Can you work these out from the model? Positions are in its coordinate system, mm. A direction names the side the tool comes from. Round coordinates to 2 decimals unless told otherwise and drop trailing zeros. Loops run counter-clockwise (first coordinate to the right, second up) from the corner with the lowest first, then second, coordinate; pieces in that order, holes last.
from build123d import *

# Parameters (mm, degrees)
SKETCH_R        = 11.1
PAD_DEPTH       = 18
SKETCH001_R     = 12
PAD001_DEPTH    = 1
SKETCH002_R     = 12
PAD002_DEPTH    = 1
SKETCH003_R     = 8
POCKET_DEPTH    = 20.001
SKETCH004_W     = 70
SKETCH004_H     = 1
POCKET001_DEPTH = 17.9
CHAMFER_SIZE    = 0.89


with BuildPart() as part:
    # Sketch → Pad (new body)
    with BuildSketch(Plane.XY):
        Circle(SKETCH_R)
    extrude(amount=PAD_DEPTH)

    # Sketch001 → Pad001 (new body)
    with BuildSketch(Plane.XY.offset(18)):
        Circle(SKETCH001_R)
    extrude(amount=PAD001_DEPTH)

    # Sketch002 → Pad002 (new body)
    with BuildSketch(Plane(origin=(0, 0, 0), x_dir=(1, 0, 0), z_dir=(0, 0, -1))):
        Circle(SKETCH002_R)
    extrude(amount=PAD002_DEPTH)

    # Sketch003 → Pocket (cut, through all)
    with BuildSketch(Plane.XY.offset(19)):
        with Locations((2, 0)):
            Circle(SKETCH003_R)
    extrude(amount=-POCKET_DEPTH, mode=Mode.SUBTRACT)

    # Sketch004 → Pocket001 (cut)
    with BuildSketch(Plane(origin=(0, 0, -1), x_dir=(1, 0, 0), z_dir=(0, 0, -1))):
        Rectangle(SKETCH004_W, SKETCH004_H)
    extrude(amount=-POCKET001_DEPTH, mode=Mode.SUBTRACT)

    # Chamfer
    chamfer_edges = [part.edges().sort_by_distance(p)[0] for p in [
        (0, -12, 0),
        (0, 12, 0),
        (-12, 0, 18),
    ]]
    chamfer(chamfer_edges, length=CHAMFER_SIZE)


solid = part.part
(1) Will these pins go through, and if not, where does the flat tip stop? P1, Ø10, axis at y = 5, z = 12.5, coming from the -X side; P2, Ø5, axis at x = -9, z = 11, coming from the +Y side; P3, Ø5, axis at x = -7, z = 12.5, coming from the +Y side.
Worked answers:
P1: stops at x = -11.09
P2: stops at y = 9
P3: stops at y = 10.15
(2) If we mould it in two halves opening along Z, with no side actions, what happens to faces 1 (the flat face through (-9, -0.5, 8)), 2 (the flat face through (-9, 0, 16.9)), 3 (the conical face through (0.24, -11.25, -0.14))? For each: released by +Z, released by -Z, zero draft, split by the parting line, or undercut.
Worked answers:
face 1: zero draft
face 2: released by -Z
face 3: undercut
(3) If we section it at D-D, the plane z = 17.5: List the corners of the cut face in (x, y) for me.
Worked answers:
outline: circle Ø22.2 at (0, 0); hole circle Ø16 at (2, 0)
(4) For faces 4 (the flat face through (-9, 0.5, 8)), 5 (the cylindrical face through (10.6, 3.3, 8.9)), 6 (the conical face through (-0.24, 11.26, -0.15)), which set-ups out of +Z, -Z, +X, -X, +Y, -Y let a thin tool reach every point of the face, with its end or its side?
Worked answers:
face 4: -Z, +X, -X
face 5: none
face 6: +Y
(5) If I drill on line 1 (X direction, y = 2, z = 1.25); line 2 (Y direction, x = 2, z = 7); line 3 (Y direction, x = 5.5, z = 7.75), over which ranges is the centre line in solid material (lowest first)?
Worked answers:
line 1: x = -10.92 to -5.75, 9.75 to 10.92
line 2: y = -10.92 to -8, 8 to 10.92
line 3: y = -9.64 to -7.19, 7.19 to 9.64
